Here's how the part is built. I have some questions about the finished solid (model axes, mm). Give positions to 0.01 mm unless a question says otherwise; leave off trailing zeros. Loops run counter-clockwise (first coordinate to the right, second up) from the corner with the lowest first, then second, coordinate; pieces in that order, holes last. Notation, with made-up numbers: (-1, 14) - (55, 14) arc R26 cw to (55, 34) - close; hole circle Ø9 at (63, 49.25). An arc over 180 degrees is marked (long way). Put each result on its own line as item: value. Start each with the question number.
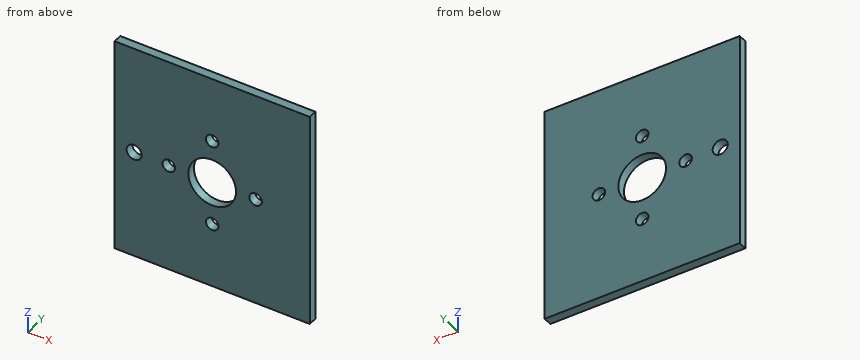
from build123d import *

# Parameters (mm, degrees)
ESQUISSE1_W                  = 90
ESQUISSE1_H                  = 100
BOSS_EXTRU_1_DEPTH           = 4
ENL_V_MAT_EXTRU_1_DEPTH      = 1401.799142477
ENL_V_MAT_EXTRU_1_DEPTH_BACK = 1401.799142477
ESQUISSE2_R                  = 11
D_GAGEMENT_M51_D             = 5.8
D_GAGEMENT_M51_DEPTH         = 20
D_GAGEMENT_M51_TIP           = 1.742495795
D_GAGEMENT_M61_D             = 7
D_GAGEMENT_M61_DEPTH         = 20
D_GAGEMENT_M61_TIP           = 2.103012167


with BuildPart() as part:
    # Esquisse1 → Boss.-Extru.1 (new body)
    with BuildSketch(Plane(origin=(0, 0, 0), x_dir=(1, 0, 0), z_dir=(0, 1, 0))):
        Rectangle(ESQUISSE1_W, ESQUISSE1_H)
    extrude(amount=BOSS_EXTRU_1_DEPTH)

    # Esquisse2 → Enlèv. mat.-Extru.1 (cut, two sides: drawn at the far end of the back side and taken through both)
    with BuildSketch(Plane(origin=(-1346.410161514, -150, 0), x_dir=(0, 0, -1), z_dir=(0, 1, 0)).offset(-ENL_V_MAT_EXTRU_1_DEPTH_BACK)):
        with Locations((0, -1346.410161514)):
            Circle(ESQUISSE2_R)
    extrude(amount=ENL_V_MAT_EXTRU_1_DEPTH + ENL_V_MAT_EXTRU_1_DEPTH_BACK, mode=Mode.SUBTRACT)

    # Dégagement M51
    with Locations(Plane(origin=(0, -8, 0), x_dir=(-1, 0, 0), z_dir=(0, -1, 0))):
        with Locations((20, 0), (0, -20), (-20, 0), (0, 20)):
            Hole(D_GAGEMENT_M51_D / 2, depth=D_GAGEMENT_M51_DEPTH)
            with Locations((0, 0, -(D_GAGEMENT_M51_DEPTH + D_GAGEMENT_M51_TIP / 2))):  # 118° drill point
                Cone(0, D_GAGEMENT_M51_D / 2, D_GAGEMENT_M51_TIP, mode=Mode.SUBTRACT)

    # Dégagement M61
    with Locations(Plane(origin=(0, 0, 0), x_dir=(-1, 0, 0), z_dir=(0, -1, 0))):
        with Locations((36, 0)):
            Hole(D_GAGEMENT_M61_D / 2, depth=D_GAGEMENT_M61_DEPTH)
            with Locations((0, 0, -(D_GAGEMENT_M61_DEPTH + D_GAGEMENT_M61_TIP / 2))):  # 118° drill point
                Cone(0, D_GAGEMENT_M61_D / 2, D_GAGEMENT_M61_TIP, mode=Mode.SUBTRACT)


solid = part.part
1) Suppose I cut it at A-A on z = 0. Please give me the cut outline in (x, y), plus the area to 3 significant figures.
2) I need wall thicknesses on line 1 (Z direction, x = -20, y = 3.1); line 2 (X direction, y = 1.4, z = -20); line 3 (X direction, y = 1.9, z = -0.5). Which ranges of each line are inside material? Lowest first, please.
3) I'm going to push flat-ended pins straight in: P1, Ø5, axis at x = -20, z = 0, coming from the +Y side; P2, Ø4, axis at x = -12, z = -38, coming from the -Y side. Where does each tip first touch, or does it pass through?
4) Suppose I cut it at C-C on y = 3.35. Please give me the cut outline in (x, z).
5) Suppose I cut it at B-B on x = -36. Please give me the cut outline in (y, z), plus the area to 3 significant figures.
6) Suppose I cut it at D-D on z = -20. Please give me the cut outline in (x, y).
Ans:
1. outline: (-45, 0) - (-39.5, 0) - (-39.5, 4) - (-45, 4) - close; (-32.5, 0) - (-22.9, 0) - (-22.9, 4) - (-32.5, 4) - close; (-17.1, 0) - (-11, 0) - (-11, 4) - (-17.1, 4) - close; (11, 0) - (17.1, 0) - (17.1, 4) - (11, 4) - close; (22.9, 0) - (45, 0) - (45, 4) - (22.9, 4) - close
1. area: 198 mm²
2. line 1: z = -50 to -2.9, 2.9 to 50
2. line 2: x = -45 to -2.9, 2.9 to 45
2. line 3: x = -45 to -39.46, -32.54 to -22.86, -17.14 to -10.99, 10.99 to 17.14, 22.86 to 45
3. P1: passes through
3. P2: stops at y = 0
4. outline: (-45, -50) - (45, -50) - (45, 50) - (-45, 50) - close; hole circle Ø7 at (-36, 0); hole circle Ø5.8 at (-20, 0); hole circle Ø22 at (0, 0); hole circle Ø5.8 at (0, -20); hole circle Ø5.8 at (0, 20); hole circle Ø5.8 at (20, 0)
5. outline: (0, -50) - (4, -50) - (4, -3.5) - (0, -3.5) - close; (0, 3.5) - (4, 3.5) - (4, 50) - (0, 50) - close
5. area: 372 mm²
6. outline: (-45, 0) - (-2.9, 0) - (-2.9, 4) - (-45, 4) - close; (2.9, 0) - (45, 0) - (45, 4) - (2.9, 4) - close
